```python
from build123d import *

# Parameters (mm, degrees)
F0_R     = 50
F0_R_2   = 45
F1_DEPTH = 50
F0_R_3   = 40
F2_DEPTH = 500
F3_DEPTH = 5
F4_R     = 10


with BuildPart() as f1:
    # F0 (on Top) → F1 (new body)
    with BuildSketch(Plane.XY):
        Circle(F0_R)
        Circle(F0_R_2, mode=Mode.SUBTRACT)
    extrude(amount=F1_DEPTH)

    # F0 (on Top) → F2 (join)
    with BuildSketch(Plane.XY):
        Circle(F0_R_2)
        Circle(F0_R_3, mode=Mode.SUBTRACT)
    extrude(amount=F2_DEPTH)

    # F0 (on Top) → F3 (join)
    with BuildSketch(Plane.XY):
        Circle(F0_R)
        Circle(F0_R_2, mode=Mode.SUBTRACT)
        Circle(F0_R_2)
        Circle(F0_R_3, mode=Mode.SUBTRACT)
        Circle(F0_R_3)
    extrude(amount=-F3_DEPTH)

    # F4
    f4_edges = [f1.edges().sort_by_distance(p)[0] for p in [
        (-50, 0, -5),
    ]]
    fillet(f4_edges, radius=F4_R)


solid = f1.part
```
Check sheet for the modelled part. Datum: model origin and axes. Units: mm. A direction names the side the tool comes from. Round coordinates to 2 decimals unless told otherwise and drop trailing zeros. Order: outer loops, then holes, each group sorted by start corner. A loop starts at its lowest first (then second) coordinate and runs counter-clockwise, first axis right, second up. Notation, with made-up numbers: (39.25, 46) - (65.25, 46) arc R26 ccw to (65.25, 65) - close; hole circle Ø7 at (-6.5, 63). An arc over 180 degrees is marked (long way). Write item = value, one per line.
Q1. Draft check along X on faces 1 (the face through (-1, 1, -5)), 2 (the face through (47.69, 15.02, 27.82)), 3 (the face through (-8.67, -39.05, 246.5)). Enter one of: pulls with the +X half, pulls with the -X half, needs draft (parallel to the pull), parting line crosses it, or undercut.
Computed:
face_1 = needs draft
face_2 = parting line crosses it
face_3 = undercut
Q2. Thickness scan on line 1 along Y through (x, z) = (-1, 268.5); line 2 along Z through (x, y) = (27.5, -22.5); line 3 along X through (y, z) = (3.5, 174.5). Record the ranges inside material, lowest first.
Computed:
line_1 = -44.99 to -39.99, 39.99 to 44.99
line_2 = -5 to 0
line_3 = -44.86 to -39.85, 39.85 to 44.86
Q3. Section check C-C (z = 261). Record the boundary of the cut face in (x, y).
Computed:
outline = circle Ø90 at (0, 0); hole circle Ø80 at (0, 0)
Q4. Go/stop test with flat-tipped pins: pin 1 (4 mm diameter, centred on x = 18, y = 25, fed in from +Z); pin 2 (4 mm diameter, centred on x = 27, z = 133, fed in from -Y); pin 3 (8 mm diameter, centred on y = 16.5, z = 347.5, fed in from +X). Record where each tip stops, or that it passes through.
Computed:
pin_1 = 0
pin_2 = -37.42
pin_3 = 43.23
Q5. Section check A-A (y = 0). Record the boundary of the cut face in (x, z), and give its area (3 significant figures).
Computed:
outline = (-50, 5) arc R10 ccw to (-40, -5) - (40, -5) arc R10 ccw to (50, 5) - (50, 50) - (45, 50) - (45, 500) - (40, 500) - (40, 0) - (-40, 0) - (-40, 500) - (-45, 500) - (-45, 50) - (-50, 50) - close
area = 5,960 mm^2
Q6. Tool access check on faces 4 (the face through (-30.2, -26.5, 500)), 5 (the face through (-1, 1, 0)). Record the directions out of +Z, -Z, +X, -X, +Y, -Y that give a thin tool (end or side, any length) a straight path to the whole face; none if there is none.
Computed:
face_4 = +Z, +X, -X, +Y, -Y
face_5 = +Z
